```python
from build123d import *

# Parameters (mm, degrees)
BOSS_EXTRUDE1_DEPTH = 25
CUT_EXTRUDE1_REACH  = 1392.455
SKETCH2_R           = 600


with BuildPart() as part:
    # Sketch1 → Boss-Extrude1 (new body)
    with BuildSketch(Plane(origin=(0, 0, 0), x_dir=(1, 0, 0), z_dir=(0, 1, 0))):
        Polygon((438.317943801, 934.970880832), (590.549562699, 847.079914683), (1028.8675065, 87.89096615), (1028.8675065, -87.89096615), (590.549562699, -847.079914683), (438.317943801, -934.970880832), (-438.317943801, -934.970880832), (-590.549562699, -847.079914683), (-1028.8675065, -87.89096615), (-1028.8675065, 87.89096615), (-590.549562699, 847.079914683), (-438.317943801, 934.970880832), align=None)
    extrude(amount=BOSS_EXTRUDE1_DEPTH)

    # Sketch2 → Cut-Extrude1 (cut, up to next)
    with BuildSketch(Plane(origin=(0, 25, 0), x_dir=(1, 0, 0), z_dir=(0, 1, 0)), mode=Mode.PRIVATE) as cut_extrude1_sk1:
        with Locations(Location((0, 0, 0), (0, 0, 270))):
            Circle(SKETCH2_R)
    cut_extrude1_tool1 = extrude(cut_extrude1_sk1.sketch, amount=-CUT_EXTRUDE1_REACH, mode=Mode.PRIVATE) & part.part
    add(cut_extrude1_tool1.solids().sort_by_distance((0, 25, 0))[0], mode=Mode.SUBTRACT)


solid = part.part
```
Design review of the part built by this model. Coordinates are the model's own, in mm. Coordinates: 2 decimals unless noted, no trailing zeros. Order: outer loops, then holes, each group sorted by start corner. A loop starts at its lowest first (then second) coordinate and runs counter-clockwise, first axis right, second up. Notation, with made-up numbers: M 88,58.5 L 115,58.5 A19 cw 115,62.5 Z; hole C -1,61.25 d7. An arc over 180 degrees is marked long. Answer as a JSON object with one key per item and string values. Group by question number.
1) For pin 1 (12 mm diameter, centred on x = -523, y = 15.5, fed in from -Z); pin 2 (1.5 mm diameter, centred on y = 14, z = -240.5, fed in from -X); pin 3 (10 mm diameter, centred on y = 3.5, z = 191.5, fed in from -X), all flat-tipped, find the tip position at first contact; note any pin that passes through.
2) Add section A-A, the plane x = 0. Write out the cut boundary in (y, z), then the cut area to 3 significant figures.
3) Add section D-D, the plane x = 722. Write out the cut boundary in (y, z).
4) Mouldability with a two-part tool opening along Z and no side actions: class faces 1 (the flat face through (-806.64, 12.32, 472.8)), 2 (the cylindrical face through (-365.09, 12.68, -476.14)), 3 (the flat face through (-812.777, 12.325, -462.171)) as pulls with the +Z half, pulls with the -Z half, needs draft (parallel to the pull), parting line crosses it, or undercut.
5) Add section C-C, the plane y = 21. Write out the cut boundary in (x, z).
6) Add section B-B, the plane z = 0. Write out the cut boundary in (x, y).
7) Wall thickness on L1, parallel to X at y = 12, z = 0; L2, parallel to Z at x = -96, y = 19.5; L3, parallel to X at y = 17.5, z = 311: over which ranges is each line inside the solid? List them lowest first.
Computed values:
{
 "1": {"pin 1": "stops at z = -889.54", "pin 2": "stops at x = -941.19", "pin 3": "stops at x = -971.94"},
 "2": {"outline": "M 0,-934.97 L 25,-934.97 L 25,-600 L 0,-600 Z; M 0,600 L 25,600 L 25,934.97 L 0,934.97 Z", "area": "16,700 mm^2"},
 "3": {"outline": "M 0,-619.4 L 25,-619.4 L 25,619.4 L 0,619.4 Z"},
 "4": {"face 1": "pulls with the +Z half", "face 2": "undercut", "face 3": "pulls with the -Z half"},
 "5": {"outline": "M -1028.87,-87.89 L -590.55,-847.08 L -438.32,-934.97 L 438.32,-934.97 L 590.55,-847.08 L 1028.87,-87.89 L 1028.87,87.89 L 590.55,847.08 L 438.32,934.97 L -438.32,934.97 L -590.55,847.08 L -1028.87,87.89 Z; hole C 0,0 d1200"},
 "6": {"outline": "M -1028.87,0 L -600,0 L -600,25 L -1028.87,25 Z; M 600,0 L 1028.87,0 L 1028.87,25 L 600,25 Z"},
 "7": {"L1": "x = -1028.87 to -600, 600 to 1028.87", "L2": "z = -934.97 to -592.27, 592.27 to 934.97", "L3": "x = -900.06 to -513.11, 513.11 to 900.06"}
}
